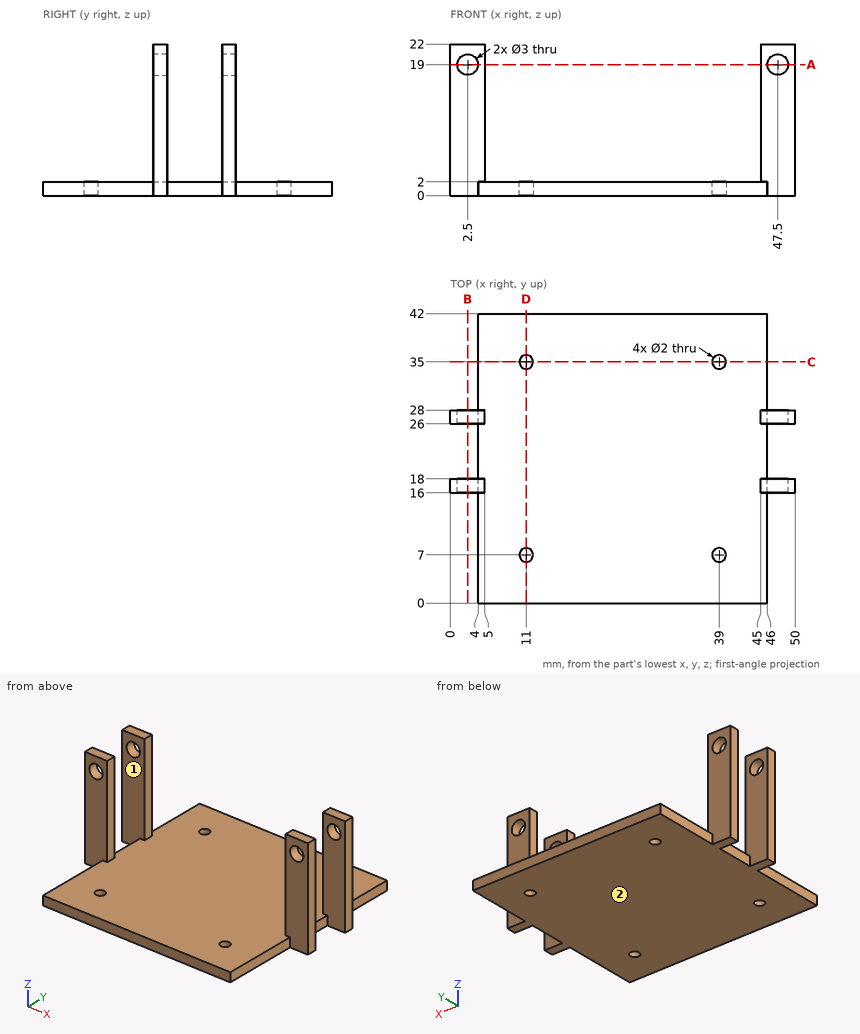
Here's the drawing with two shaded views (mm, measured from the low corner). I have some questions. Coordinates: 2 decimals unless noted, no trailing zeros. Order: outer loops, then holes, each group sorted by start corner. A loop starts at its lowest first (then second) coordinate and runs counter-clockwise, first axis right, second up. Notation, with made-up numbers: M 33.25,78 L 49.25,78 A21 cw 49.25,112 Z; hole C 63,55.5 d11. An arc over 180 degrees is marked long. Write item = value, one per line.
(1) Suppose I cut it at D-D on x = 11. Please give me the cut outline in (y, z), plus the area to 3 significant figures.
Results are:
outline = M 0,0 L 6,0 L 6,2 L 0,2 Z; M 8,0 L 34,0 L 34,2 L 8,2 Z; M 36,0 L 42,0 L 42,2 L 36,2 Z
area = 76.0 mm2
(2) I need wall thicknesses on line 1 along Y through (x, z) = (39, 1.4); line 2 along X through (y, z) = (26.85, 19); line 3 along X through (y, z) = (35, 0.85). Which ranges of each line are inside material? Lowest first, please. Write a range as [from, to].
Results are:
line_1 = [0, 6], [8, 34], [36, 42]
line_2 = [0, 1], [4, 5], [45, 46], [49, 50]
line_3 = [4, 10], [12, 38], [40, 46]
(3) Suppose I cut it at C-C on y = 35. Please give me the cut outline in (x, z), plus the area to 3 significant figures.
Results are:
outline = M 4,0 L 10,0 L 10,2 L 4,2 Z; M 12,0 L 38,0 L 38,2 L 12,2 Z; M 40,0 L 46,0 L 46,2 L 40,2 Z
area = 76.0 mm2
(4) Suppose I cut it at A-A on z = 19. State how many separate pieces and enclosed holes the cut face has, plus the area to 3 significant figures.
Results are:
separate_pieces = 8
enclosed_holes = 0
area = 16.0 mm2
(5) If we mould it in two halves opening along Y, with no side actions, what happens to the marked faces 1 and 2? For each: pulls with the +Y half, pulls with the -Y half, needs draft (parallel to the pull), parting line crosses it, or undercut.
Results are:
face_1 = undercut
face_2 = needs draft
(6) Suppose I cut it at B-B on x = 2.5. Please give me the cut outline in (y, z), plus the area to 3 significant figures.
Results are:
outline = M 16,0 L 18,0 L 18,17.5 L 16,17.5 Z; M 16,20.5 L 18,20.5 L 18,22 L 16,22 Z; M 26,0 L 28,0 L 28,17.5 L 26,17.5 Z; M 26,20.5 L 28,20.5 L 28,22 L 26,22 Z
area = 76.0 mm2
(7) For pin 1 Ø0.6 at (y, z) = (8.5, 0.5) entering from -X; pin 2 Ø3 at (x, y) = (11, 35) entering from +Z; pin 3 Ø5.5 at (x, z) = (48, 10) entering from -Y, each with a flat end and sliding along its axis, tell me the tip position at first contact or that it passes through.
Results are:
pin_1 = 4
pin_2 = 2
pin_3 = 16
